The figure shows three views and two pictorial views of one solid part (mm, origin at its lowest corner). Answer the questions. Round coordinates to 2 decimals unless told otherwise and drop trailing zeros. Order: outer loops, then holes, each group sorted by start corner. A loop starts at its lowest first (then second) coordinate and runs counter-clockwise, first axis right, second up. Notation, with made-up numbers: (-19.5, 73.25) - (30.5, 73.25) arc R11 cw to (30.5, 93.25) - close; hole circle Ø3 at (-26, -5.5). An arc over 180 degrees is marked (long way). Write item = value, one per line.
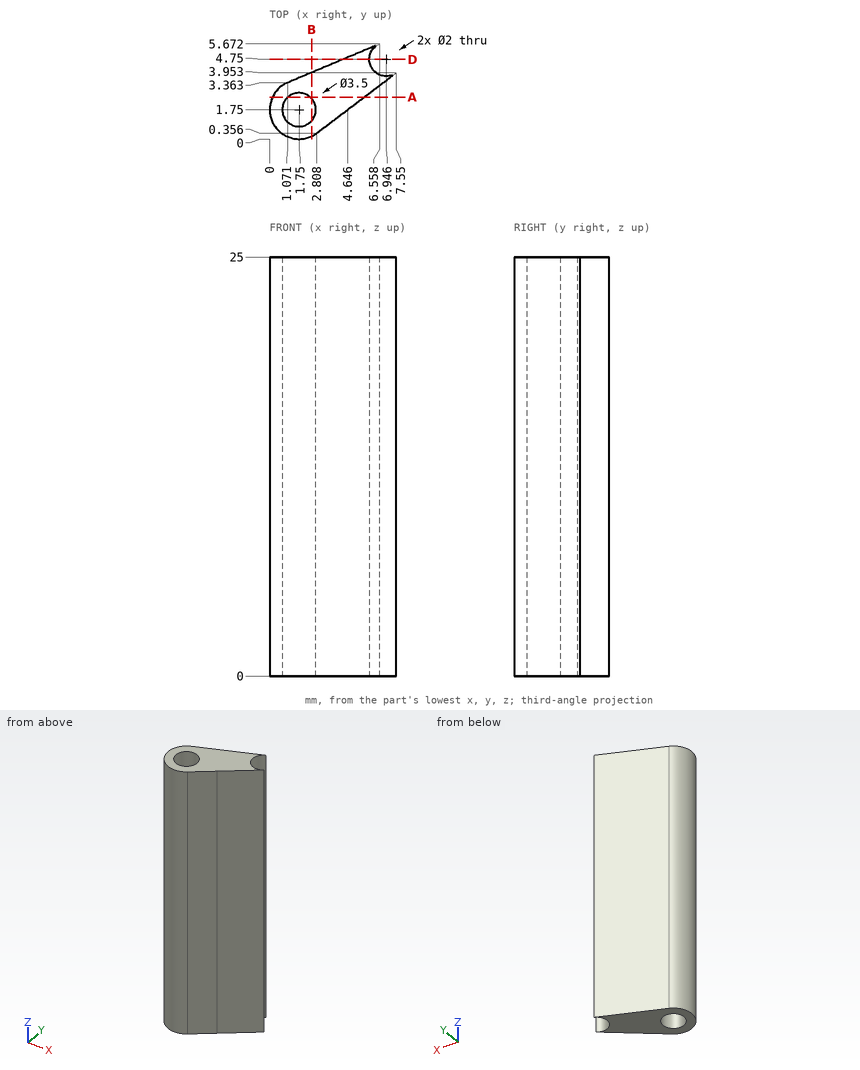
Q1. Section D-D on y = 4.75 is taken. Determine the outline of the cut face in (x, z).
Model answer:
outline = (4.37, 0) - (5.95, 0) - (5.95, 25) - (4.37, 25) - close
Q2. Section A-A on y = 2.5 is taken. Determine the outline of the cut face in (x, z) (1 decimal).
Model answer:
outline = (0.2, 0) - (1.1, 0) - (1.1, 25) - (0.2, 25) - close; (2.4, 0) - (5.6, 0) - (5.6, 25) - (2.4, 25) - close
Q3. Find the intervals of material crossed by line 1 (Y direction, x = 1.5, z = 8.5) (1 decimal); line 2 (Y direction, x = 1.75, z = 1.5); line 3 (X direction, y = 2.3, z = 11.5) (1 decimal), in increasing order. Write a range as from..to.
Model answer:
line_1 = 0..0.8, 2.7..3.5
line_2 = 0..0.75, 2.75..3.65
line_3 = 0.1..0.9, 2.6..5.4
Q4. Section B-B on x = 2.5 is taken. Determine the outline of the cut face in (y, z) (1 decimal).
Model answer:
outline = (0.2, 0) - (1.1, 0) - (1.1, 25) - (0.2, 25) - close; (2.4, 0) - (4, 0) - (4, 25) - (2.4, 25) - close
Q5. Flat-ended cylindrical pins translate along their axes: P1, Ø3, axis at x = 1.5, z = 4.5, coming from the +Y side (1 decimal); P2, Ø1.5, axis at y = 4.5, z = 13, coming from the -X side; P3, Ø1.8, axis at x = 6.95, y = 4.75, coming from the -Z side. Find the tip coordinate at first contact, or state that the pin passes through.
Model answer:
P1 = 4.2
P2 = 1.99
P3 = through
